Verification items for this drawing (mm, ordinates from the low corner). A direction names the side the tool comes from. Coordinates: 2 decimals unless noted, no trailing zeros. Order: outer loops, then holes, each group sorted by start corner. A loop starts at its lowest first (then second) coordinate and runs counter-clockwise, first axis right, second up. Notation, with made-up numbers: (37.5, 77) -> (63.5, 77) arc R20 cw to (63.5, 99) -> close; hole circle Ø4 at (31, 40). An arc over 180 degrees is marked (long way). Put each result on its own line as item: value. Start each with the question number.
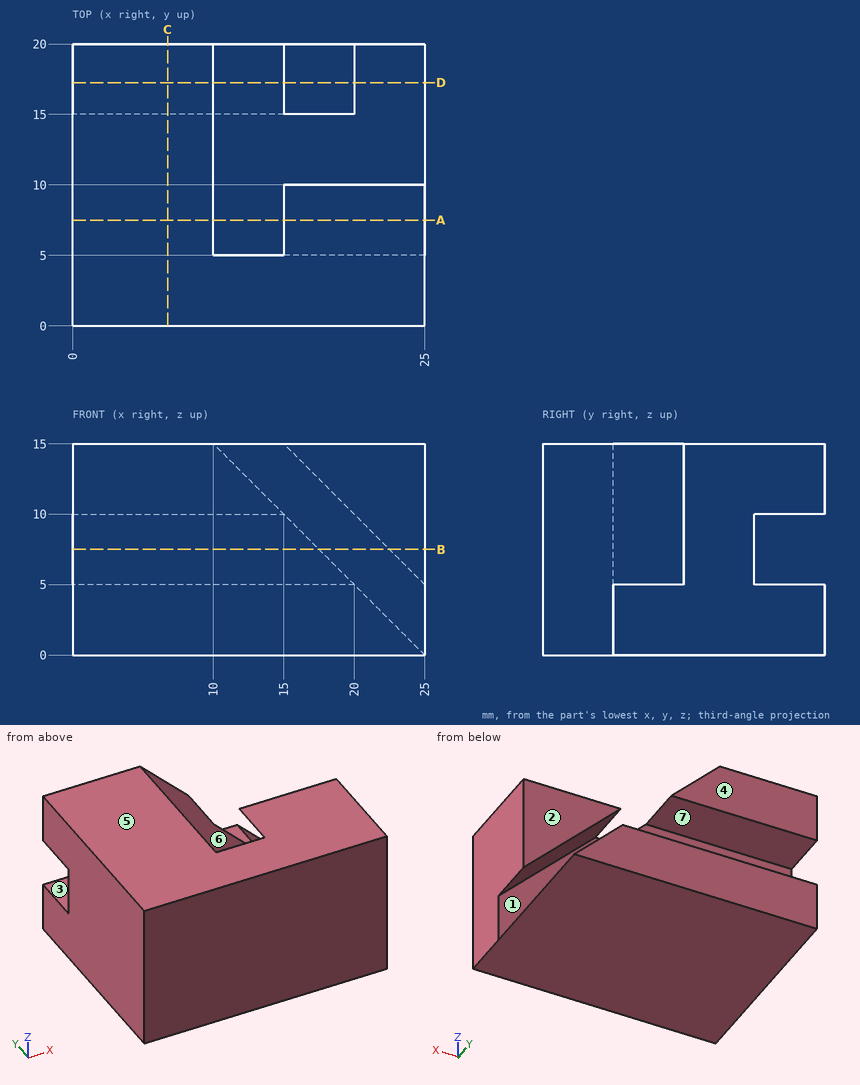
1) Mould release check, pull along Z, two halves, no side actions. Record for the marked faces 4, 5, 6 and 7: +Z half, -Z half, draft (parallel to the pull), parting line (faces both ways), or undercut.
2) Access from +Z, -Z, +X, -X, +Y, -Y to the whole of each face (thin tool, end or side, straight path). Record for the marked faces 1, 2 and 3.
3) Sectioned sample at B-B (z = 7.5). Record the boundary of the cut face in (x, y), plus the area to 4 significant figures.
4) Gauge pin test, flat end, axial feed: pin 1 (3 mm diameter, centred on x = 20, z = 9, fed in from +Y). Record the tip position at first contact, or that the pin passes through.
5) Sectioned sample at C-C (x = 6.75). Record the boundary of the cut face in (y, z), plus the area to 3 significant figures.
6) Sectioned sample at D-D (y = 17.25). Record the boundary of the cut face in (x, z).
7) Scan lines: line 1 along Z through (x, y) = (2, 18); line 2 along Y through (x, z) = (10.5, 14.75); line 3 along Y through (x, z) = (8, 8.5). Record each from-to range of solid material in increasing order. Write a range as [from, to].
8) Sectioned sample at A-A (y = 7.5). Record the boundary of the cut face in (x, z).
Entries:
1. face 4: draft
1. face 5: +Z half
1. face 6: undercut
1. face 7: undercut
2. face 1: +Y
2. face 2: +Z, +X, +Y
2. face 3: +X, -X, +Y
3. outline: (0, 0) -> (25, 0) -> (25, 10) -> (22.5, 10) -> (22.5, 5) -> (17.5, 5) -> (17.5, 15) -> (0, 15) -> close
3. area: 312.5 mm2
4. pin 1: stops at y = 10
5. outline: (0, 0) -> (20, 0) -> (20, 5) -> (15, 5) -> (15, 10) -> (20, 10) -> (20, 15) -> (0, 15) -> close
5. area: 275 mm2
6. outline: (0, 0) -> (25, 0) -> (20, 5) -> (0, 5) -> close; (0, 10) -> (15, 10) -> (10, 15) -> (0, 15) -> close
7. line 1: z = [0, 5], [10, 15]
7. line 2: y = [0, 5]
7. line 3: y = [0, 15]
8. outline: (0, 0) -> (25, 0) -> (10, 15) -> (0, 15) -> close; (15, 15) -> (25, 5) -> (25, 15) -> close
